```python
from build123d import *

# Parameters (mm, degrees)
SKETCH1_R               = 8
SKETCH1_R_2             = 6
BOSS_EXTRUDE1_DEPTH     = 168
CUT_EXTRUDE1_DEPTH      = 169.380521439
CUT_EXTRUDE1_DEPTH_BACK = 169.380521439
SKETCH2_R               = 4.5
CUT_EXTRUDE2_DEPTH      = 169.380521548
CUT_EXTRUDE2_DEPTH_BACK = 169.380521548
SKETCH3_R               = 1.5
CUT_EXTRUDE3_DEPTH      = 169.38052155
CUT_EXTRUDE3_DEPTH_BACK = 169.38052155
SKETCH4_R               = 2


with BuildPart() as part:
    # Sketch1 → Boss-Extrude1 (new, symmetric)
    with BuildSketch(Plane(origin=(0, 0, 0), x_dir=(1, 0, 0), z_dir=(0, 1, 0))):
        with Locations(Location((0, 0, 0), (0, 0, 90))):
            Circle(SKETCH1_R)
        with Locations(Location((0, 0, 0), (0, 0, 90))):
            Circle(SKETCH1_R_2, mode=Mode.SUBTRACT)
    extrude(amount=BOSS_EXTRUDE1_DEPTH, both=True)

    # Sketch2 → Cut-Extrude1 (cut, two sides: drawn at the far end of the back side and taken through both)
    with BuildSketch(Plane(origin=(0, 0, 0), x_dir=(0, 0, -1), z_dir=(1, 0, 0)).offset(-CUT_EXTRUDE1_DEPTH_BACK)):
        Circle(SKETCH2_R)
    extrude(amount=CUT_EXTRUDE1_DEPTH + CUT_EXTRUDE1_DEPTH_BACK, mode=Mode.SUBTRACT)

    # Sketch3 → Cut-Extrude2 (cut, two sides: drawn at the far end of the back side and taken through both)
    with BuildSketch(Plane.XY.offset(-CUT_EXTRUDE2_DEPTH_BACK)):
        Circle(SKETCH3_R)
    extrude(amount=CUT_EXTRUDE2_DEPTH + CUT_EXTRUDE2_DEPTH_BACK, mode=Mode.SUBTRACT)

    # Sketch4 → Cut-Extrude3 (cut, two sides: drawn at the far end of the back side and taken through both)
    with BuildSketch(Plane.XY.offset(-CUT_EXTRUDE3_DEPTH_BACK)):
        with Locations((0, 159)):
            Circle(SKETCH4_R)
        with Locations((0, -159)):
            Circle(SKETCH4_R)
    extrude(amount=CUT_EXTRUDE3_DEPTH + CUT_EXTRUDE3_DEPTH_BACK, mode=Mode.SUBTRACT)


solid = part.part
```
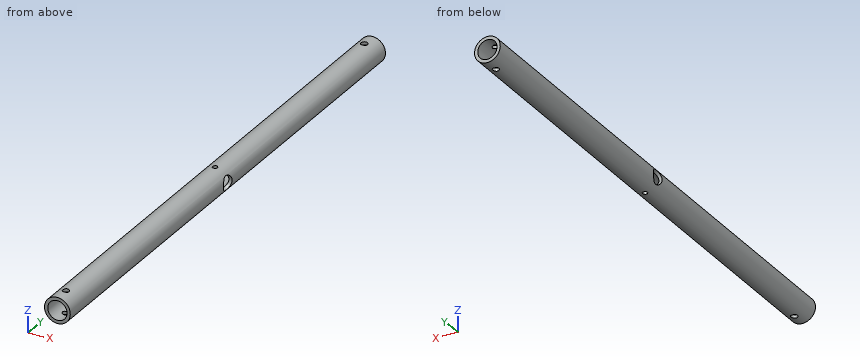
Here's how the part is built. I have some questions about the finished solid (model axes, mm). Coordinates: 2 decimals unless noted, no trailing zeros. Loops run counter-clockwise (first coordinate to the right, second up) from the corner with the lowest first, then second, coordinate; pieces in that order, holes last. Notation, with made-up numbers: (43.25, -34) -> (92.25, -34) arc R16 cw to (92.25, -12) -> close; hole circle Ø10 at (-5.75, 55.5). An arc over 180 degrees is marked (long way). Return JSON: item names as keys, results as strings.
1) I need wall thicknesses on line 1 (Y direction, x = 0, z = 6.5); line 2 (Z direction, x = 0.5, y = 64.5). Which ranges of each line are inside material? Lowest first, please. Write a range as from..to.
Results below:
{"line 1": "-168..-161, -157..-1.5, 1.5..157, 161..168", "line 2": "-7.98..-5.98, 5.98..7.98"}
2) Will these pins go through, and if not, where does the flat tip stop? pin 1 (3.5 mm diameter, centred on x = 0, y = -159, fed in from +Z); pin 2 (5 mm diameter, centred on y = -99.5, z = 5.5, fed in from -X); pin 3 (4 mm diameter, centred on x = -6, y = 34, fed in from +Z).
Results below:
{"pin 1": "through", "pin 2": "x = -7.42", "pin 3": "z = 6.93"}
3) If we section it at A-A, the plane z = 0: Write out the boundary of the cut face in (x, y), then the cut area to 3 significant figures.
Results below:
{"outline": "(-8, -168) -> (-6, -168) -> (-6, -4.5) -> (-8, -4.5) -> close; (-8, 4.5) -> (-6, 4.5) -> (-6, 168) -> (-8, 168) -> close; (6, -168) -> (8, -168) -> (8, -4.5) -> (6, -4.5) -> close; (6, 4.5) -> (8, 4.5) -> (8, 168) -> (6, 168) -> close", "area": "1,310 mm²"}
4) If we section it at B-B, the plane y = -117: Write out the boundary of the cut face in (x, z).
Results below:
{"outline": "circle Ø16 at (0, 0); hole circle Ø12 at (0, 0)"}
